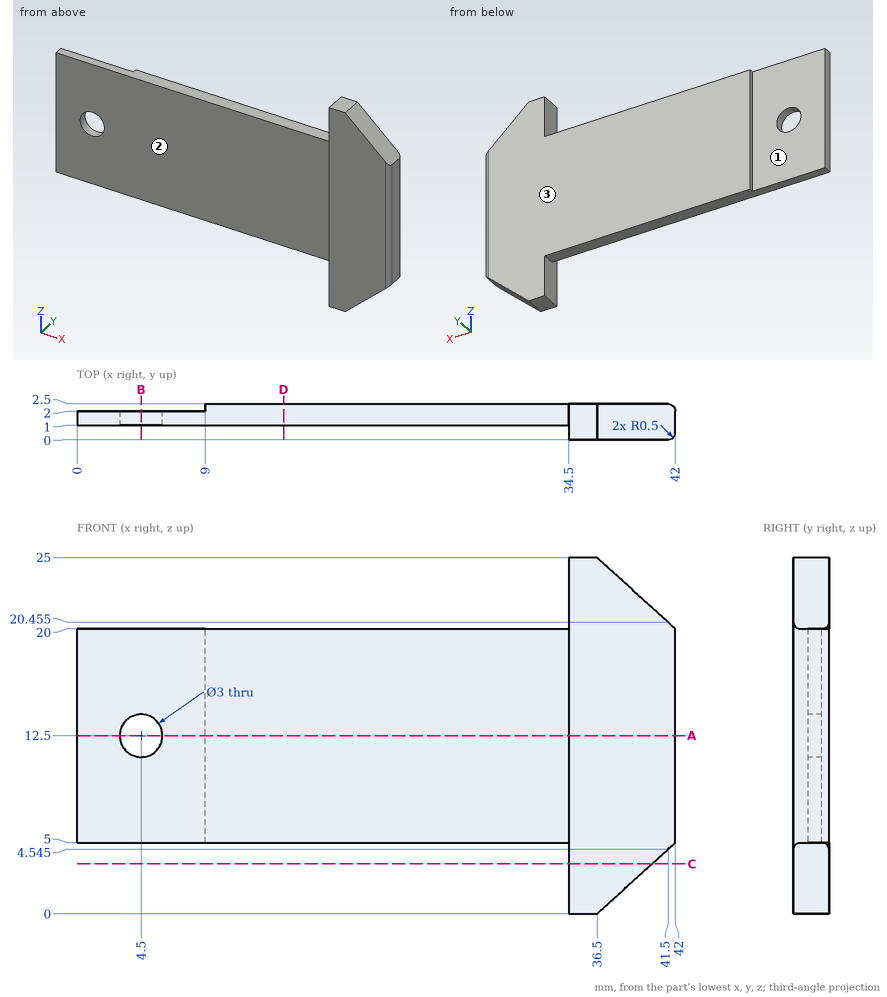
Check sheet for the drawn part. Datum: minimum x, y, z corner. Units: mm. A direction names the side the tool comes from. Round coordinates to 2 decimals unless told otherwise and drop trailing zeros. Loops run counter-clockwise (first coordinate to the right, second up) from the corner with the lowest first, then second, coordinate; pieces in that order, holes last. Notation, with made-up numbers: (69.25, -22.75) - (77.25, -22.75) arc R20 ccw to (77.25, -3.75) - close; hole circle Ø7 at (-0.75, 48.5). An arc over 180 degrees is marked (long way). Write each question's results on one line, items separated by ' | '. Start each with the question number.
Q1. Gauge pin test, flat ends, axial feed: P1, Ø12, axis at x = 17, z = 17, coming from the -Y side; P2, Ø1.5, axis at y = 1, z = 12, coming from the -X side; P3, Ø5, axis at x = 4.5, z = 12.5, coming from the +Y side; P4, Ø0.6, axis at y = 2.5, z = 9, coming from the -X side. Record the tip position at first contact, or that the pin passes through.
Q2. Cross-section at C-C on z = 3.5. Enter the section's corners in (x, y).
Q3. Cross-section at D-D on x = 14.5. Enter the section's corners in (y, z).
Q4. Cross-section at B-B on x = 4.5. Enter the section's corners in (y, z).
Q5. Access from +Z, -Z, +X, -X, +Y, -Y to the whole of each face (thin tool, end or side, straight path). Record for the marked faces 1, 2 and 3.
Q6. Cross-section at A-A on z = 12.5. Enter the section's corners in (x, y).
Q7. Thickness scan on line 1 (Z direction, x = 4.5, y = 1.7); line 2 (Y direction, x = 20.5, z = 13.5); line 3 (Z direction, x = 27, y = 2). Record the ranges inside material, lowest first. Write a range as [from, to].
Answers below:
1) P1: stops at y = 1 | P2: stops at x = 0 | P3: stops at y = 2 | P4: stops at x = 9
2) outline: (34.5, 0) - (40.35, 0) - (40.35, 2.5) - (34.5, 2.5) - close
3) outline: (1, 5) - (2.5, 5) - (2.5, 20) - (1, 20) - close
4) outline: (1, 5) - (2, 5) - (2, 11) - (1, 11) - close; (1, 14) - (2, 14) - (2, 20) - (1, 20) - close
5) face 1: +Z, -Z, -X, +Y | face 2: +Z, -Z, -X, -Y | face 3: +Z, -Z, +X, -X, +Y
6) outline: (0, 1) - (3, 1) - (3, 2) - (0, 2) - close; (6, 1) - (34.5, 1) - (34.5, 0) - (41.5, 0) arc R0.5 ccw to (42, 0.5) - (42, 2) arc R0.5 ccw to (41.5, 2.5) - (9, 2.5) - (9, 2) - (6, 2) - close
7) line 1: z = [5, 11], [14, 20] | line 2: y = [1, 2.5] | line 3: z = [5, 20]
